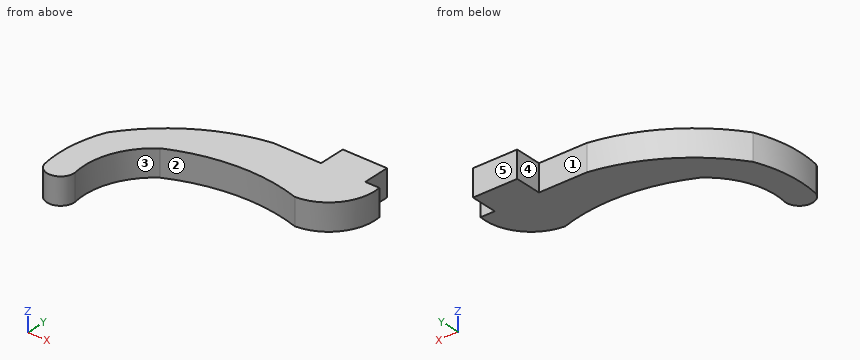
```python
from build123d import *

# Parameters (mm, degrees)
BOSS_EXTRUDE1_DEPTH = 1.524


with BuildPart() as part:
    # Sketch1 → Boss-Extrude1 (new body)
    with BuildSketch(Plane.XY):
        with BuildLine():
            Line((-111.845658384, 0), (-111.845658384, -1.524))
            Line((-111.845658384, -1.524), (-114.602460127, -1.524))
            ThreePointArc((-114.602460127, -1.524), (-118.141425353, -2.883409348), (-120.878346422, -5.506676721))
            ThreePointArc((-120.878346422, -5.506676721), (-121.373374596, -7.40819224), (-121.311747708, -9.372121029))
            ThreePointArc((-121.311747708, -9.372121029), (-120.420802234, -9.907256069), (-119.785228435, -9.084942689))
            ThreePointArc((-119.785228435, -9.084942689), (-119.570544838, -6.84579555), (-118.193770427, -5.066930411))
            ThreePointArc((-118.193770427, -5.066930411), (-114.602460127, -4.096166999), (-110.905453841, -4.510938975))
            ThreePointArc((-110.905453841, -4.510938975), (-109.055147034, -3.538155103), (-108.49557312, -1.524))
            Line((-108.49557312, -1.524), (-109.305658384, -1.524))
            Line((-109.305658384, -1.524), (-109.305658384, 0))
            Line((-109.305658384, 0), (-111.845658384, 0))
        make_face()
    extrude(amount=BOSS_EXTRUDE1_DEPTH)


solid = part.part
```
Can you work these out from the model? Positions are in its coordinate system, mm. Face numbers are marked on the shaded views. A direction names the side the tool comes from. Coordinates: 2 decimals unless noted, no trailing zeros. Loops run counter-clockwise (first coordinate to the right, second up) from the corner with the lowest first, then second, coordinate; pieces in that order, holes last.
Item 1: Suppose I cut it at B-B (y = -8.5). Please give me the cut outline in (x, z).
Answers below:
outline: (-121.41, 0) - (-119.85, 0) - (-119.85, 1.52) - (-121.41, 1.52) - close
Item 2: If we mould it in two halves opening along Y, with no side actions, what happens to the marked faces 3, 4 and 5? For each: released by +Y, released by -Y, zero draft, split by the parting line, or undercut.
Answers below:
face 3: undercut
face 4: zero draft
face 5: released by +Y
Item 3: Please list where these lines run through material, in increasing order: L1, parallel to X at y = -1, z = 0.15; L2, parallel to Y at x = -113.75, z = 0.7; L3, parallel to Y at x = -119.5, z = 0.15.
Answers below:
L1: x = -111.85 to -109.31
L2: y = -4.07 to -1.52
L3: y = -6.68 to -3.93
Item 4: Suppose I cut it at C-C (x = -120.5). Please give me the cut outline in (y, z), then the cut area to 3 significant figures.
Answers below:
outline: (-9.92, 0) - (-5, 0) - (-5, 1.52) - (-9.92, 1.52) - close
area: 7.50 mm2
Item 5: I'm going to push flat-ended pins straight in: pin 1 (0.5 mm diameter, centred on y = -0.5, z = 1, fed in from -X); pin 2 (0.8 mm diameter, centred on x = -112.5, z = 0.5, fed in from +Y). Where does each tip first touch, or does it pass through?
Answers below:
pin 1: stops at x = -111.85
pin 2: stops at y = -1.52
Item 6: Suppose I cut it at A-A (z = 0.8). Please give me the cut outline in (x, y), then the cut area to 3 significant figures.
Answers below:
outline: (-121.31, -9.37) arc R0.78 ccw to (-119.79, -9.08) arc R4.05 cw to (-118.19, -5.07) arc R9.96 cw to (-110.91, -4.51) arc R2.63 ccw to (-108.5, -1.52) - (-109.31, -1.52) - (-109.31, 0) - (-111.85, 0) - (-111.85, -1.52) - (-114.6, -1.52) arc R9.6 ccw to (-120.88, -5.51) arc R6.89 ccw to start
area: 39.0 mm2
Item 7: Which directions (+Z, -Z, +X, -X, +Y, -Y) give clear straight access to the entire face, cutting with the end or side of a thin tool? Please do the marked faces 1 and 2.
Answers below:
face 1: +Z, -Z, -X, +Y
face 2: +Z, -Z, -Y
